CAD build for the part. Positions are in the model's coordinates, mm. Coordinates: 2 decimals unless noted, no trailing zeros. Loops run counter-clockwise (first coordinate to the right, second up) from the corner with the lowest first, then second, coordinate; pieces in that order, holes last. Notation, with made-up numbers: (-33.75, 85.25) -> (-5.75, 85.25) arc R21 cw to (-5.75, 120.25) -> close; hole circle Ø1 at (38.5, 48). An arc over 180 degrees is marked (long way). Answer as a JSON object with one key per item and string values. Group by question number.
from build123d import *

# Parameters (mm, degrees)
F0_R     = 20
F1_DEPTH = 5
F2_R     = 14
F3_DEPTH = 5
F5_D     = 12.2
F6_SIZE  = 1


with BuildPart() as f1:
    # F0 (on Top) → F1 (new body)
    with BuildSketch(Plane.XY):
        Circle(F0_R)
    extrude(amount=F1_DEPTH)

    # F2 (on face) → F3 (join)
    with BuildSketch(Plane.XY.offset(5)):
        Circle(F2_R)
    extrude(amount=F3_DEPTH)

    # F5 (through all)
    with Locations(Plane(origin=(0, 0, 0), x_dir=(1, 0, 0), z_dir=(0, 0, -1))):
        with Locations((0, 0)):
            Hole(F5_D / 2)

    # F6
    f6_edges = [f1.edges().sort_by_distance(p)[0] for p in [
        (-14, 0, 10),
    ]]
    chamfer(f6_edges, length=F6_SIZE)


solid = f1.part
Item 1: Band-saw the part on D-D, the plane x = 16. List the corners of the cut face in (y, z).
Item 2: Drill centre lines: L1, parallel to Y at x = 0, z = 5.5; L2, parallel to Y at x = 0, z = 2; L3, parallel to Z at x = 3, y = -17. Where is each one in solid material? Low to high.
Item 3: Pull direction X, two halves, no side cores. Call faces 1 (the cylindrical face through (12.932, -5.362, 6.972)), 2 (the cylindrical face through (6.094, -0.268, 5.07)), 3 (the flat face through (-14, -4, 5)): +X half, -X half, draft (parallel to the pull), parting line (faces both ways), or undercut.
Item 4: Flat gauge pins, fed straight in: P1, Ø1, axis at y = 14, z = 5, coming from the -X side; P2, Ø2, axis at y = -12.5, z = 4, coming from the +X side; P3, Ø1, axis at x = -4, y = -5.5, coming from the -Z side; P4, Ø4, axis at y = 14, z = 5.5, coming from the -X side. Where does each tip first touch, or does it go through?
Item 5: Band-saw the part on C-C, the plane z = 5.5. List the corners of the cut face in (x, y), and give its area (3 significant figures).
Item 6: Band-saw the part on A-A, the plane x = 0. List the corners of the cut face in (y, z), and give its area (3 significant figures).
Reply:
{
 "1": {"outline": "(-12, 0) -> (12, 0) -> (12, 5) -> (-12, 5) -> close"},
 "2": {"L1": "-14 to -6.1, 6.1 to 14", "L2": "-20 to -6.1, 6.1 to 20", "L3": "0 to 5"},
 "3": {"face 1": "parting line", "face 2": "undercut", "face 3": "draft"},
 "4": {"P1": "x = -14.76", "P2": "x = 16.36", "P3": "z = 0", "P4": "x = -15.95"},
 "5": {"outline": "circle Ø28 at (0, 0); hole circle Ø12.2 at (0, 0)", "area": "499 mm²"},
 "6": {"outline": "(-20, 0) -> (-6.1, 0) -> (-6.1, 10) -> (-13, 10) -> (-14, 9) -> (-14, 5) -> (-20, 5) -> close; (6.1, 0) -> (20, 0) -> (20, 5) -> (14, 5) -> (14, 9) -> (13, 10) -> (6.1, 10) -> close", "area": "217 mm²"}
}
